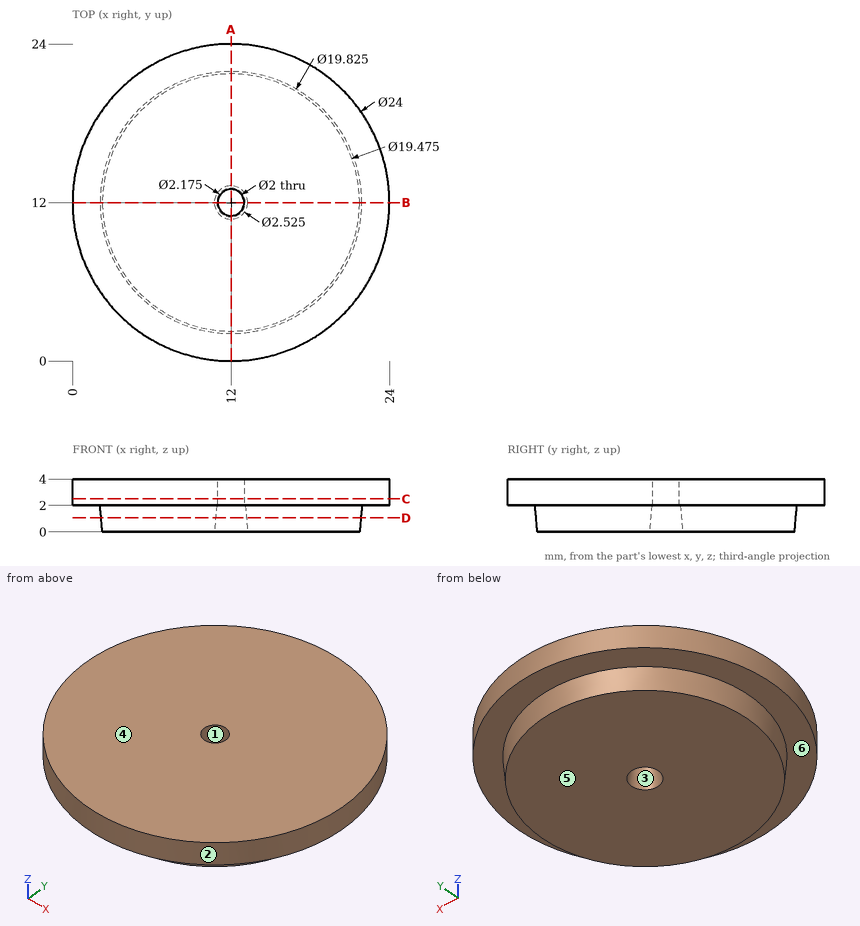
Source: three-view drawing plus pictorial views. Frame: mm from the lowest corner of the part. A direction names the side the tool comes from. Round coordinates to 2 decimals unless told otherwise and drop trailing zeros. Order: outer loops, then holes, each group sorted by start corner. A loop starts at its lowest first (then second) coordinate and runs counter-clockwise, first axis right, second up. Notation, with made-up numbers: (10, 28) -> (31, 28) arc R20 cw to (31, 41) -> close; hole circle Ø9 at (-9.5, -17.75). An arc over 180 degrees is marked (long way). Use CSV: the item, a comma, the result in double quotes. Start each with the question number.
1) Draft query along X for the marked faces 1, 2, 3 and 4. Return one class per face: +X half, -X half, draft (parallel to the pull), parting line (faces both ways), or undercut.
2) Section C-C (z = 2.5). Return the cut outline in (x, y).
3) Section A-A (x = 12). Return the cut outline in (y, z), and give its area (3 significant figures).
4) Section D-D (z = 1.05). Return the cut outline in (x, y), and give its area (3 significant figures).
5) Material intervals for line 1 along Y through (x, z) = (12, 2.9); line 2 along Z through (x, y) = (11, 1); line 3 along Y through (x, z) = (14.5, 2.55), sorted ascending. Write a range as from..to.
6) Set-up query: the marked faces 5 and 6. Return all of +Z, -Z, +X, -X, +Y, -Y with unobstructed straight access to the full face (end or side cutting, diameter ignored); none if empty.
7) First-contact query: pin 1 Ø1.5 at (y, z) = (21, 3.5) entering from -X; pin 2 Ø2 at (y, z) = (8, 2) entering from -X; pin 3 Ø1 at (y, z) = (18, 2.5) entering from -X; pin 4 Ø0.7 at (x, y) = (12.5, 12) entering from -Z. Flat tips, straight axial feed; report the tip coordinate or a pass-through.
Returned:
1,face 1,"undercut"
1,face 2,"parting line"
1,face 3,"undercut"
1,face 4,"draft"
2,outline,"circle Ø24 at (12, 12); hole circle Ø2 at (12, 12)"
3,outline,"(0, 2) -> (2.09, 2) -> (2.26, 0) -> (10.74, 0) -> (10.91, 2) -> (11, 2) -> (11, 4) -> (0, 4) -> close; (13, 2) -> (13.09, 2) -> (13.26, 0) -> (21.74, 0) -> (21.91, 2) -> (24, 2) -> (24, 4) -> (13, 4) -> close"
3,area,"78.6 mm²"
4,outline,"circle Ø19.66 at (12, 12); hole circle Ø2.34 at (12, 12)"
4,area,"299 mm²"
5,line 1,"y = 0..11, 13..24"
5,line 2,"z = 2..4"
5,line 3,"y = 0.26..23.74"
6,face 5,"-Z, +X, -X, +Y, -Y"
6,face 6,"-Z"
7,pin 1,"stops at x = 3.29"
7,pin 2,"stops at x = 0.38"
7,pin 3,"stops at x = 1.33"
7,pin 4,"passes through"
